Design review of the part shown in the three views and the two pictorial views. Dimensions are in mm from the part's minimum x, y and z. Coordinates: 2 decimals unless noted, no trailing zeros. Order: outer loops, then holes, each group sorted by start corner. A loop starts at its lowest first (then second) coordinate and runs counter-clockwise, first axis right, second up. Notation, with made-up numbers: M 43.5,50.25 L 60.5,50.25 A32 cw 60.5,87.25 Z; hole C 15.5,12 d2. An arc over 180 degrees is marked long. Use CSV: the item, a comma, the result in double quotes.
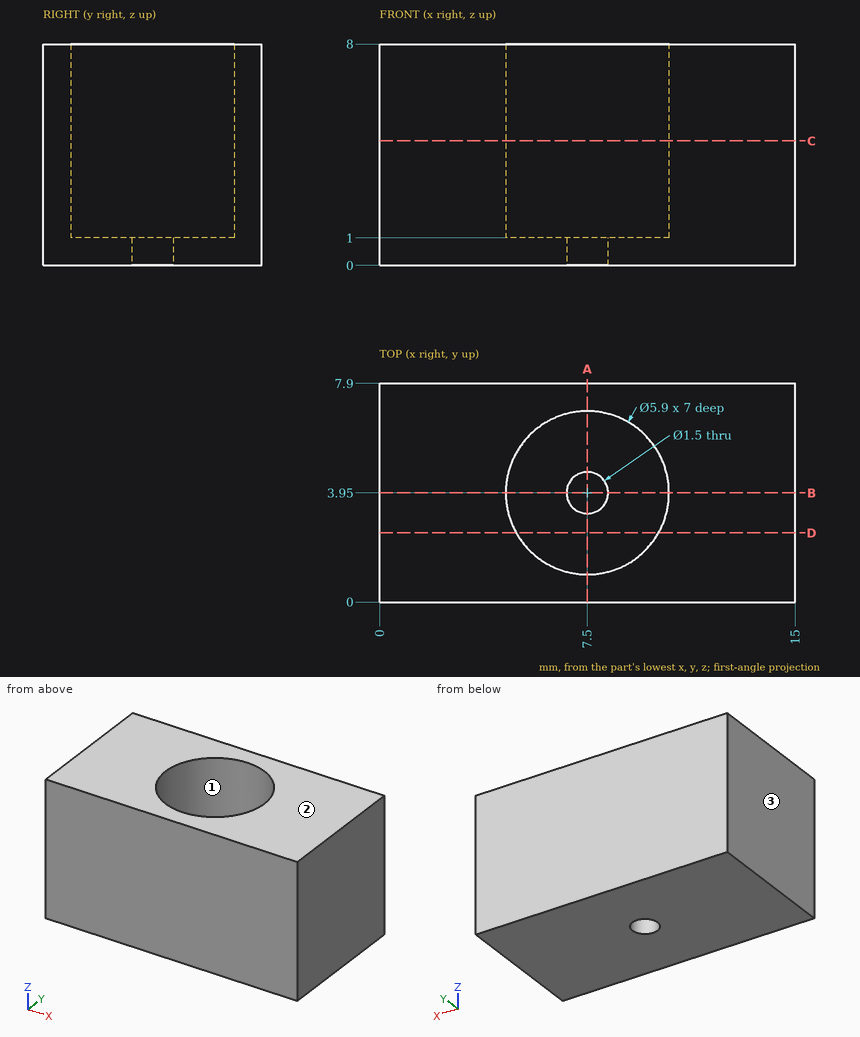
(1) Wall thickness on probe 1 along Y at (x, z) = (7.5, 0.7); probe 2 along Y at (x, z) = (7.5, 6); probe 3 along X at (y, z) = (2.25, 3): over which ranges is each line inside the solid? List them lowest first.
The answers:
probe 1,"y = 0 to 3.2, 4.7 to 7.9"
probe 2,"y = 0 to 1, 6.9 to 7.9"
probe 3,"x = 0 to 5.09, 9.91 to 15"
(2) Add section C-C on z = 4.5. State the section outline as (x, y) points, and give its area (3 significant figures).
The answers:
outline,"M 0,0 L 15,0 L 15,7.9 L 0,7.9 Z; hole C 7.5,3.95 d5.9"
area,"91.2 mm2"
(3) Add section A-A on x = 7.5. State the section outline as (y, z) points, and give its area (3 significant figures).
The answers:
outline,"M 0,0 L 3.2,0 L 3.2,1 L 1,1 L 1,8 L 0,8 Z; M 4.7,0 L 7.9,0 L 7.9,8 L 6.9,8 L 6.9,1 L 4.7,1 Z"
area,"20.4 mm2"
(4) Add section D-D on y = 2.5. State the section outline as (x, z) points.
The answers:
outline,"M 0,0 L 15,0 L 15,8 L 10.07,8 L 10.07,1 L 4.93,1 L 4.93,8 L 0,8 Z"
(5) Add section B-B on y = 3.95. State the section outline as (x, z) points.
The answers:
outline,"M 0,0 L 6.75,0 L 6.75,1 L 4.55,1 L 4.55,8 L 0,8 Z; M 8.25,0 L 15,0 L 15,8 L 10.45,8 L 10.45,1 L 8.25,1 Z"
(6) Clearance check with flat-ended pins moving along their axes: P1, Ø3, axis at x = 8, y = 3.5, coming from the +Z side; P2, Ø1.5, axis at y = 6.5, z = 5.5, coming from the -X side. State where each tip first meets the part, or that it passes through.
The answers:
P1,"stops at z = 1"
P2,"stops at x = 0"
(7) The part is to be moulded in two halves that separate along X. For the marked faces 1, 2 and 3, say which applies: pulls with the +X half, pulls with the -X half, needs draft (parallel to the pull), parting line crosses it, or undercut.
The answers:
face 1,"undercut"
face 2,"needs draft"
face 3,"pulls with the -X half"
